CAD build for the part. Positions are in the model's coordinates, mm. A direction names the side the tool comes from. Round coordinates to 2 decimals unless told otherwise and drop trailing zeros. Loops run counter-clockwise (first coordinate to the right, second up) from the corner with the lowest first, then second, coordinate; pieces in that order, holes last. Notation, with made-up numbers: M 61,-36 L 81,-36 A24 ccw 81,-1 Z; hole C 37,87.25 d3. An arc over 180 degrees is marked long. Put each result on its own line as item: value. Start each with the question number.
Autodesk Inventor part; units mm, degrees
ref_plane "Work Plane2" through (0, 0, 0) normal (0.7071068, 0, -0.7071068) x (0, -1, 0)
ref_plane "Work Plane3" through (0, 0, 0) normal (-0.7071068, 0, -0.7071068) x (0, 1, 0)
ref_plane "YZ Plane" through (0, 0, 0) normal (1, 0, 0) x (0, 1, 0)
sketch "Sketch1" plane through (0, 0, 0) normal (0, 0, 1) x (1, 0, 0)
  line L0 (-26, 14.5) -> (26, 14.5)
  line L1 (26, 14.5) -> (26, -14.5)
  line L2 (26, -14.5) -> (-26, -14.5)
  line L3 (-26, -14.5) -> (-26, 14.5)
  line L4 (-26, 14.5) -> (26, -14.5) construction
  line L5 (26, 14.5) -> (-26, -14.5) construction
  point P0 (0, 0)
  dimension "d0" = 52
  dimension "d1" = 29
extrude "Extrusion1" add sketch "Sketch1" along normal blind 4
sketch "Sketch2" plane through (0, 0, 4) normal (0, 0, 1) x (1, 0, 0)
  line L0 (-21.1, 8.1) -> (21.1, 8.1)
  line L1 (21.1, 8.1) -> (21.1, -8.1)
  line L2 (21.1, -8.1) -> (-21.1, -8.1)
  line L3 (-21.1, -8.1) -> (-21.1, 8.1)
  line L4 (-21.1, 8.1) -> (21.1, -8.1) construction
  line L5 (21.1, 8.1) -> (-21.1, -8.1) construction
  point P0 (0, 0)
  dimension "d4" = 42.2
  dimension "d5" = 16.2
hole "Hole1" at (-21.1, 8.1, 4) at (21.1, 8.1, 4) at (21.1, -8.1, 4) at (-21.1, -8.1, 4) direction (0, 0, -1) diameter 5 end through all
ref_plane "Work Plane1" through (0, -14.5, 0) normal (1, 0, 0) x (0, 0, -1)
ref_plane "Work Plane2" through (0, 0, 0) normal (0.7071068, 0, -0.7071068) x (0, -1, 0)
ref_plane "Work Plane3" through (0, 0, 0) normal (-0.7071068, 0, -0.7071068) x (0, 1, 0)
sketch "Sketch4" plane through (0, 0, 0) normal (-0.7071068, 0, -0.7071068) x (0, 1, 0)
  line L0 (14.5, 15.5563) -> (14.5, -21.2132)
  line L1 (14.5, 0) -> (-25.5, 0)
  line L2 (-25.5, 0) -> (-25.5, 20)
  line L3 (-25.5, 20) -> (14.5, 20)
  line L4 (14.5, 20) -> (14.5, 0)
  point P0 (0, 0)
  dimension "d14" = 40
  dimension "d15" = 20
extrude "Extrusion2" add sketch "Sketch4" against normal blind 5.5
sketch "Sketch5" plane through (0, 0, 0) normal (0.7071068, 0, -0.7071068) x (0, -1, 0)
  line L0 (-14.5, -21.2132) -> (-14.5, 15.5563)
  line L1 (-14.5, 0) -> (25.5, 0)
  line L2 (25.5, 0) -> (25.5, 20)
  line L3 (25.5, 20) -> (-14.5, 20)
  line L4 (-14.5, 20) -> (-14.5, 0)
  point P0 (0, 0)
  dimension "d18" = 40
  dimension "d19" = 20
extrude "Extrusion3" add sketch "Sketch5" against normal blind 5.5
sketch "Sketch7" plane through (0, 0, 0) normal (-0.7071068, 0, -0.7071068) x (-0.7071068, 0, 0.7071068)
  line L0 (-20, 14.5) -> (0, 14.5)
  line L1 (-13, 14.5) -> (-13, -25.5)
  line L2 (0, -25.5) -> (-20, -25.5)
  line L3 (-7, 14.5) -> (-7, -25.5)
  line L4 (-20, -25.5) -> (-20, 14.5)
  line L5 (-13, 14.5) -> (-7, 14.5)
  line L6 (-13, -25.5) -> (-7, -25.5)
  point P0 (0, 0)
  dimension "d22" = 7
  dimension "d23" = 13
extrude "Extrusion4" add sketch "Sketch7" along normal blind 1.5 contours L0 L3 L2 L1
sketch "Sketch8" plane through (-26, -14.5, 4) normal (0, -1, 0) x (1, 0, 0)
  line L0 (22.1109, -0.1109) -> (26, -4)
  line L1 (26, -4) -> (29.8891, -0.1109)
  line L2 (29.8891, -0.1109) -> (29.8891, 0)
  line L3 (0, 0) -> (52, 0)
  line L4 (22.1109, -0.1109) -> (26, -4)
  line L5 (22.1109, -0.1109) -> (22.1109, 0)
  line L6 (22.1109, 0) -> (29.8891, 0)
extrude "Extrusion5" add sketch "Sketch8" along normal blind 11
sketch "Sketch9" plane through (-1.0607, 0, -1.0607) normal (-0.7071068, 0, -0.7071068) x (-0.7071068, 0, 0.7071068)
  line L0 (-13, -25.5) -> (-7, -25.5)
  line L1 (-20, -25.5) -> (-20, 14.5)
  point P0 (0, 0)
  point P1 (-10, -20)
  dimension "d28" = 5.5
  dimension "d29" = 10
hole "Hole2" at (6.0104, -20, -8.1317) direction (0.7071068, 0, 0.7071068) diameter 5.5 end through all counterbore diameter 10 counterbore depth 1.5
sketch "Sketch10" plane through (0, 0, 0) normal (0.7071068, 0, -0.7071068) x (-0.7071068, 0, -0.7071068)
  line L0 (20, -25.5) -> (20, 14.5)
  line L1 (0, -25.5) -> (20, -25.5)
  point P0 (0, 0)
  point P1 (10, -20)
  dimension "d37" = 10
  dimension "d38" = 5.5
hole "Hole3" at (-7.0711, -20, -7.0711) direction (-0.7071068, 0, 0.7071068) diameter 5.5 end through all
properties part number "Estrutura - suporteCam"
(1) Cut at D-D on z = 2. List the corners of the cut face in (x, y).
(2) Cut at C-C on z = -12.5. List the corners of the cut face in (x, y), and give its area (3 significant figures).
(3) Cut at B-B on x = -21.1. List the corners of the cut face in (y, z).
(4) Drill centre lines: line 1 along Y through (x, z) = (21.1, 1.8); line 2 along X through (y, z) = (8.1, 2.55); line 3 along X through (y, z) = (10, 3.25). Where is each one in solid material? Low to high.
(5) Tool access for faces 1 (the flat face through (-17, 0, 0)), 2 (the flat face through (-15, -14.5, 2)), 3 (the flat face through (6.04, -25.24, -8.16)), 4 (the flat face through (15, -14.5, 2)), 5 (the cylindrical face through (6.6, -15, -7.6)): list every direction of +Z, -Z, +X, -X, +Y, -Y with a clear straight run to the whole face (end or side of a thin tool).
(6) Cut at A-A on y = 8.1. List the corners of the cut face in (x, z), and give its area (3 significant figures).
(7) Flat gauge pins, fed straight in: pin 1 Ø6 at (x, y) = (21.1, -8.1) entering from +Z; pin 2 Ø6 at (x, y) = (-2, -10) entering from -Z; pin 3 Ø8 at (x, y) = (-3, -4) entering from -Z; pin 4 Ø4 at (x, y) = (21.1, 8.1) entering from +Z. Where does each tip first touch, or does it go through?
(8) Mould opens along Z. For faces 6 (the flat face through (0, 14.5, 0.4)), 7 (the flat face through (16.059, -5.78, -12.225)), 8 (the flat face through (17, 0, 0)) say: +Z half, -Z half, draft (parallel to the pull), parting line (faces both ways), or undercut.
Taken from the geometry:
1. outline: M -26,-14.5 L -5.78,-14.5 L -5.78,-25.5 L 5.78,-25.5 L 5.78,-14.5 L 26,-14.5 L 26,14.5 L -26,14.5 Z; hole C -21.1,-8.1 d5; hole C -21.1,8.1 d5; hole C 21.1,-8.1 d5; hole C 21.1,8.1 d5
2. outline: M -15.78,-25.5 L -12.5,-25.5 L -12.5,14.5 L -15.78,14.5 Z; M 12.5,-25.5 L 15.78,-25.5 L 15.78,14.5 L 12.5,14.5 Z
2. area: 263 mm2
3. outline: M -14.5,0 L -10.6,0 L -10.6,4 L -14.5,4 Z; M -5.6,0 L 5.6,0 L 5.6,4 L -5.6,4 Z; M 10.6,0 L 14.5,0 L 14.5,4 L 10.6,4 Z
4. line 1: -14.5 to -10.6, -5.6 to 5.6, 10.6 to 14.5
4. line 2: -26 to -23.6, -18.6 to 18.6, 23.6 to 26
4. line 3: -26 to -22.72, -19.48 to 19.48, 22.72 to 26
5. face 1: -X, +Y, -Y
5. face 2: +Z, -X, -Y
5. face 3: -Z, +Y, -Y
5. face 4: +Z, +X, -Y
5. face 5: none
6. outline: M -26,0 L -23.6,0 L -23.6,4 L -26,4 Z; M -18.6,0 L -7.78,0 L -18.03,-10.25 L -14.14,-14.14 L 0,0 L 4.95,-4.95 L 3.89,-6.01 L 8.13,-10.25 L 9.19,-9.19 L 14.14,-14.14 L 18.03,-10.25 L 7.78,0 L 18.6,0 L 18.6,4 L -18.6,4 Z; M 23.6,0 L 26,0 L 26,4 L 23.6,4 Z
6. area: 367 mm2
7. pin 1: z = 4
7. pin 2: z = -5
7. pin 3: z = -7
7. pin 4: through
8. face 6: draft
8. face 7: -Z half
8. face 8: undercut
